For this review, take the finished solid that the model builds, in its own axes (mm). A direction names the side the tool comes from. Give positions to 0.01 mm unless a question says otherwise; leave off trailing zeros. Order: outer loops, then holes, each group sorted by start corner. A loop starts at its lowest first (then second) coordinate and runs counter-clockwise, first axis right, second up. Notation, with made-up numbers: M 12.5,-7.5 L 39.5,-7.5 A14 cw 39.5,-2.5 Z; hole C 62,59 d8. An arc over 180 degrees is marked long. Use CSV: the item, a comma, the result in double quotes. Start each with the question number.
(1) Draft analysis for pull direction X (two halves, no side actions). For faces 1 (the face through (-17, 15.57, 3.2)), 2 (the face through (-35, -3, 3)), 3 (the face through (0, -19, 2)), 4 (the face through (35, -3, 3)), state which applies: pulls with the +X half, pulls with the -X half, needs draft (parallel to the pull), parting line crosses it, or undercut.
(2) Wall thickness on L1, parallel to X at y = 14.5, z = 2.75; L2, parallel to Y at x = -19, z = 1.5; L3, parallel to Y at x = -22, z = 5: over which ranges is each line inside the solid? List them lowest first. Write a range as from..to.
(3) Consider section A-A (x = 19). Write out the cut boundary in (y, z).
(4) Consider section D-D (y = -15.5). Write out the cut boundary in (x, z), and give its area (3 significant figures).
(5) Clearance check with flat-ended pins moving along their axes: P1, Ø8, axis at x = -17, y = -13, coming from the +Z side; P2, Ø4, axis at x = 11.5, y = -14, coming from the +Z side; P3, Ø1, axis at x = -2, z = 5.5, coming from the -Y side. State where each tip first meets the part, or that it passes through.
(6) Tool access review of faces 5 (the face through (-8, 8, 6.5)), 6 (the face through (0, -15, 4.5)): name each direction out of +Z, -Z, +X, -X, +Y, -Y from which nothing blocks a thin tool from reaching the whole face with its end or side.
(7) Consider section B-B (y = 0). Write out the cut boundary in (x, z), and give its area (3 significant figures).
(8) Consider section C-C (z = 3). Write out the cut boundary in (x, y).
```python
from build123d import *

# Parameters (mm, degrees)
F0_W     = 70
F0_H     = 38
F0_R     = 1.5
F0_R_2   = 11
F1_DEPTH = 6.5
F2_W     = 70
F2_H     = 7.9
F2_R     = 1.5
F3_DEPTH = 2
F4_R     = 5


with BuildPart() as f1:
    # F0 (on Top) → F1 (new body)
    with BuildSketch(Plane.XY):
        Rectangle(F0_W, F0_H)
        with Locations((-15.5, -15.5)):
            Circle(F0_R, mode=Mode.SUBTRACT)
        with Locations((-19, -6)):
            Circle(F0_R, mode=Mode.SUBTRACT)
        with Locations((15.5, -15.5)):
            Circle(F0_R, mode=Mode.SUBTRACT)
        with Locations((19, -6)):
            Circle(F0_R, mode=Mode.SUBTRACT)
        with Locations((-15.5, 15.5)):
            Circle(F0_R, mode=Mode.SUBTRACT)
        Circle(F0_R_2, mode=Mode.SUBTRACT)
        with Locations((15.5, 15.5)):
            Circle(F0_R, mode=Mode.SUBTRACT)
    extrude(amount=F1_DEPTH)

    # F2 (on face) → F3 (cut)
    with BuildSketch(Plane.XY.offset(6.5)):
        with Locations((0, -15.05)):
            Rectangle(F2_W, F2_H)
        with Locations((-15.5, -15.5)):
            Circle(F2_R, mode=Mode.SUBTRACT)
        with Locations((15.5, -15.5)):
            Circle(F2_R, mode=Mode.SUBTRACT)
    extrude(amount=-F3_DEPTH, mode=Mode.SUBTRACT)

    # F4
    f4_edges = [f1.edges().sort_by_distance(p)[0] for p in [
        (35, 19, 3.25),
        (-35, 19, 3.25),
    ]]
    fillet(f4_edges, radius=F4_R)


solid = f1.part
```
Check result:
1,face 1,"undercut"
1,face 2,"pulls with the -X half"
1,face 3,"needs draft"
1,face 4,"pulls with the +X half"
2,L1,"x = -34.97..-16.62, -14.38..14.38, 16.62..34.97"
2,L2,"y = -19..-7.5, -4.5..19"
2,L3,"y = -11.1..19"
3,outline,"M -19,0 L -7.5,0 L -7.5,6.5 L -11.1,6.5 L -11.1,4.5 L -19,4.5 Z; M -4.5,0 L 19,0 L 19,6.5 L -4.5,6.5 Z"
4,outline,"M -35,0 L -17,0 L -17,4.5 L -35,4.5 Z; M -14,0 L 14,0 L 14,4.5 L -14,4.5 Z; M 17,0 L 35,0 L 35,4.5 L 17,4.5 Z"
4,area,"288 mm^2"
5,P1,"stops at z = 6.5"
5,P2,"stops at z = 4.5"
5,P3,"stops at y = -11.1"
6,face 5,"+Z, +X, -X, +Y, -Y"
6,face 6,"+Z, +X, -X, -Y"
7,outline,"M -35,0 L -11,0 L -11,6.5 L -35,6.5 Z; M 11,0 L 35,0 L 35,6.5 L 11,6.5 Z"
7,area,"312 mm^2"
8,outline,"M -35,-19 L 35,-19 L 35,14 A5 ccw 30,19 L -30,19 A5 ccw -35,14 Z; hole C -19,-6 d3; hole C -15.5,-15.5 d3; hole C -15.5,15.5 d3; hole C 0,0 d22; hole C 15.5,-15.5 d3; hole C 15.5,15.5 d3; hole C 19,-6 d3"
